Can you work these out from the model? Positions are in its coordinate system, mm. Give positions to 0.01 mm unless a question says otherwise; leave off trailing zeros. Order: outer loops, then holes, each group sorted by start corner. A loop starts at its lowest first (then second) coordinate and runs counter-clockwise, first axis right, second up.
Item 1: If we mould it in two halves opening along Y, with no side actions, what happens to faces 1 (the cylindrical face through (0.14, 3.19, 0.39)), 2 (the flat face through (3, 2, 0.8)), 3 (the cylindrical face through (-0.159, 4.687, 0.394))? For each: +Y half, -Y half, draft (parallel to the pull), parting line (faces both ways), or undercut.
Item 2: If I drill on line 1 along X through (y, z) = (-4.25, 0.1); line 2 along Y through (x, z) = (-1.5, 0.45); line 3 along Y through (x, z) = (1, 0.5), over which ranges is the centre line in solid material (lowest first)?
Item 3: I'm going to push a flat-ended pin straight in: pin 1 Ø5 at (x, y) = (3.5, 0) entering from -Z. Where does the tip first touch, or does it pass through?
Item 4: I want a section at C-C, the plane z = 0.3. Write out the boundary of the cut face in (x, y), then the cut area to 3 significant figures.
Item 5: I want a section at D-D, the plane x = 0. Write out the boundary of the cut face in (y, z).
Item 6: I want a section at B-B, the plane x = 1.5. Write out the boundary of the cut face in (y, z).
Item 7: I want a section at A-A, the plane y = -3.25. Write out the boundary of the cut face in (x, z), then the cut area to 3 significant figures.
```python
from build123d import *

# Parameters (mm, degrees)
SKETCH_1_R      = 0.6
EXTRUDE_1_DEPTH = 0.8
FILLET_1_R      = 0.2


with BuildPart() as part:
    # 草图1 → 凸台-拉伸1 (new body)
    with BuildSketch(Plane.XY):
        with BuildLine():
            Line((-0.4, -3.567629953), (-0.4, -5.567629953))
            Line((-0.4, -5.567629953), (-3, -4.870962053))
            Line((-3, -4.870962053), (-3, -3.605010402))
            ThreePointArc((-3, -3.605010402), (0, 4.69), (3, -3.605010402))
            Line((3, -3.605010402), (3, -4.870962053))
            Line((3, -4.870962053), (0.4, -5.567629953))
            Line((0.4, -5.567629953), (0.4, -3.567629953))
            ThreePointArc((0.4, -3.567629953), (0, 3.191302331), (-0.4, -3.567629953))
        make_face()
        with Locations((-1.5, -4.267629953)):
            Circle(SKETCH_1_R, mode=Mode.SUBTRACT)
        with Locations((1.5, -4.267629953)):
            Circle(SKETCH_1_R, mode=Mode.SUBTRACT)
    extrude(amount=EXTRUDE_1_DEPTH)

    # 圆角1
    fillet_1_edges = [part.edges().sort_by_distance(p)[0] for p in [
        (-0.4, -5.567629953, 0.4),
        (-3, -4.870962053, 0.4),
        (-3, -3.605010402, 0.4),
        (3, -3.605010402, 0.4),
        (3, -4.870962053, 0.4),
        (0.4, -5.567629953, 0.4),
    ]]
    fillet(fillet_1_edges, radius=FILLET_1_R)


solid = part.part
```
Results list:
1. face 1: undercut
1. face 2: draft
1. face 3: parting line
2. line 1: x = -3 to -2.1, -0.9 to -0.4, 0.4 to 0.9, 2.1 to 3
2. line 2: y = -5.27 to -4.87, -3.67 to -3.24, 2.84 to 4.44
2. line 3: y = -5.41 to -4.6, -3.94 to -3.44, 3.04 to 4.58
3. pin 1: stops at z = 0
4. outline: (-3.07, -3.55) arc R0.2 cw to (-3, -3.7) - (-3, -4.72) arc R0.2 ccw to (-2.85, -4.91) - (-0.65, -5.5) arc R0.2 ccw to (-0.4, -5.31) - (-0.4, -3.57) arc R3.39 cw (long way) to (0.4, -3.57) - (0.4, -5.31) arc R0.2 ccw to (0.65, -5.5) - (2.85, -4.91) arc R0.2 ccw to (3, -4.72) - (3, -3.7) arc R0.2 cw to (3.07, -3.55) arc R4.69 ccw (long way) to start; hole circle Ø1.2 at (-1.5, -4.27); hole circle Ø1.2 at (1.5, -4.27)
4. area: 34.6 mm2
5. outline: (3.19, 0) - (4.69, 0) - (4.69, 0.8) - (3.19, 0.8) - close
6. outline: (-5.27, 0) - (-4.87, 0) - (-4.87, 0.8) - (-5.27, 0.8) - close; (-3.67, 0) - (-3.24, 0) - (-3.24, 0.8) - (-3.67, 0.8) - close; (2.84, 0) - (4.44, 0) - (4.44, 0.8) - (2.84, 0.8) - close
7. outline: (-3.38, 0) - (-1.48, 0) - (-1.48, 0.8) - (-3.38, 0.8) - close; (1.48, 0) - (3.38, 0) - (3.38, 0.8) - (1.48, 0.8) - close
7. area: 3.04 mm2
